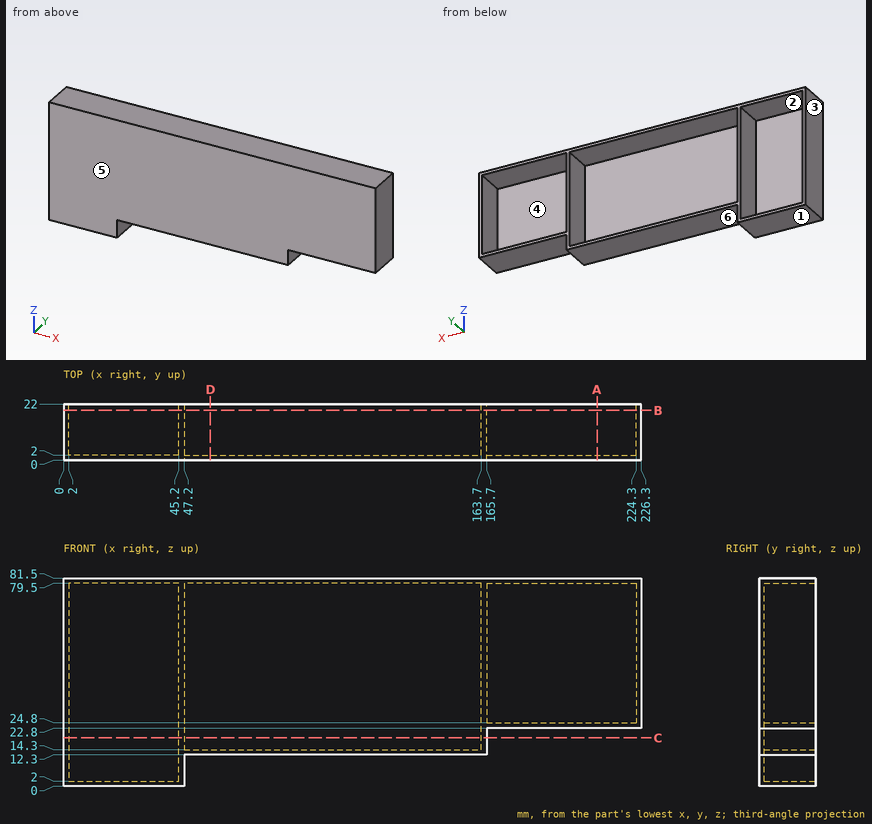
Answer from the drawing. Dimensions are ordinates in mm from the lowest x, y and z of the part. A direction names the side the tool comes from. Give positions to 0.01 mm unless a question says otherwise; leave off trailing zeros. Loops run counter-clockwise (first coordinate to the right, second up) from the corner with the lowest first, then second, coordinate; pieces in that order, holes last. Notation, with made-up numbers: M 49,10.5 L 90,10.5 A25 ccw 90,25.5 Z; hole C -28,-2 d9. An arc over 180 degrees is marked long. One line per item, written item: value.
Q1. Flat-ended cylindrical pins translate along their axes: P1, Ø2, axis at x = 101, y = 13.5, coming from the -Z side; P2, Ø5, axis at x = 127, z = 27, coming from the -Y side; P3, Ø4, axis at x = 191.5, z = 28, coming from the +Y side; P4, Ø3, axis at y = 6.5, z = 17.5, coming from the +X side. Find the tip coordinate at first contact, or state that the pin passes through.
Working result:
P1: stops at z = 12.3
P2: stops at y = 0
P3: stops at y = 2
P4: stops at x = 165.7
Q2. Find the intervals of material crossed by line 1 (X direction, y = 7.75, z = 71); line 2 (X direction, y = 14, z = 19); line 3 (X direction, y = 15.5, z = 5), in increasing order. Write a range as from..to.
Working result:
line 1: x = 0..2, 45.2..47.2, 163.7..165.7, 224.3..226.3
line 2: x = 0..2, 45.2..47.2, 163.7..165.7
line 3: x = 0..2, 45.2..47.2
Q3. A cutting plane is placed at A-A on x = 209. Determine the outline of the cut face in (y, z), then the cut area to 3 significant figures.
Working result:
outline: M 0,22.8 L 22,22.8 L 22,24.8 L 2,24.8 L 2,79.5 L 22,79.5 L 22,81.5 L 0,81.5 Z
area: 197 mm^2
Q4. A cutting plane is placed at D-D on x = 57.5. Determine the outline of the cut face in (y, z).
Working result:
outline: M 0,12.3 L 22,12.3 L 22,14.3 L 2,14.3 L 2,79.5 L 22,79.5 L 22,81.5 L 0,81.5 Z
Q5. A cutting plane is placed at C-C on z = 19. Determine the outline of the cut face in (x, y).
Working result:
outline: M 0,0 L 165.7,0 L 165.7,22 L 163.7,22 L 163.7,2 L 47.2,2 L 47.2,22 L 45.2,22 L 45.2,2 L 2,2 L 2,22 L 0,22 Z
Q6. For the marked faces 4, 5 and 6, determine the directions among +Z, -Z, +X, -X, +Y, -Y from which every point of the face is accessible in a straight line to the end or side of a thin tool.
Working result:
face 4: +Y
face 5: +Z, -Z, +X, -X, -Y
face 6: -Z, +X, +Y, -Y
Q7. A cutting plane is placed at B-B on y = 19.5. Determine the outline of the cut face in (x, z), then the cut area to 4 significant figures.
Working result:
outline: M 0,0 L 47.2,0 L 47.2,12.3 L 165.7,12.3 L 165.7,22.8 L 226.3,22.8 L 226.3,81.5 L 0,81.5 Z; hole M 2,2 L 45.2,2 L 45.2,79.5 L 2,79.5 Z; hole M 47.2,14.3 L 163.7,14.3 L 163.7,79.5 L 47.2,79.5 Z; hole M 165.7,24.8 L 224.3,24.8 L 224.3,79.5 L 165.7,79.5 Z
area: 1,455 mm^2
Q8. Determine the mould class of the marked faces 1, 2 and 3 for opening direction X: +X half, -X half, draft (parallel to the pull), parting line (faces both ways), or undercut.
Working result:
face 1: draft
face 2: undercut
face 3: -X half
